Model file for the job. Use its own axes, mm. Round coordinates to 2 decimals unless told otherwise and drop trailing zeros. Loops run counter-clockwise (first coordinate to the right, second up) from the corner with the lowest first, then second, coordinate; pieces in that order, holes last.
from build123d import *

# Parameters (mm, degrees)
SKETCH1_R           = 60.5
SKETCH1_R_2         = 2.3
BOSS_EXTRUDE1_DEPTH = 2
SKETCH3_W           = 20
SKETCH3_H           = 4.8
CUT_EXTRUDE1_DEPTH  = 5
SKETCH4_W           = 165.999999998
SKETCH4_H           = 5
CUT_EXTRUDE2_DEPTH  = 5
SKETCH5_R           = 2.1
CUT_EXTRUDE3_DEPTH  = 5
SKETCH6_W           = 30
SKETCH6_H           = 2
SKETCH6_W_2         = 150
CUT_EXTRUDE4_DEPTH  = 5
SKETCH7_R           = 2.1
CUT_EXTRUDE5_DEPTH  = 5


with BuildPart() as part:
    # Sketch1 → Boss-Extrude1 (new body)
    with BuildSketch(Plane.XY):
        Polygon((125.000000001, -69.9), (75.000000001, -69.9), (75.000000001, -71.9), (55.000000001, -71.9), (55.000000001, -69.9), (-54.999999999, -69.9), (-54.999999999, -71.9), (-74.999999999, -71.9), (-74.999999999, -69.9), (-124.999999999, -69.9), (-124.999999999, -19.9), (-126.999999999, -19.9), (-126.999999999, 0.1), (-124.999999999, 0.1), (-124.999999999, 110.1), (-126.999999999, 110.1), (-126.999999999, 130.1), (-124.999999999, 130.1), (-124.999999999, 180.1), (125.000000001, 180.1), (125.000000001, 130.1), (127.000000001, 130.1), (127.000000001, 110.1), (125.000000001, 110.1), (125.000000001, 0.1), (127.000000001, 0.1), (127.000000001, -19.9), (125.000000001, -19.9), align=None)
        Circle(SKETCH1_R, mode=Mode.SUBTRACT)
        with Locations((0, -64)):
            Circle(SKETCH1_R_2, mode=Mode.SUBTRACT)
    extrude(amount=BOSS_EXTRUDE1_DEPTH)

    # Sketch3 → Cut-Extrude1 (cut)
    with BuildSketch(Plane.XY.offset(2)):
        with Locations((-102.999999999, 88.505234687)):
            Rectangle(SKETCH3_W, SKETCH3_H)
        with Locations((-102.999999999, 73.505234687)):
            Rectangle(SKETCH3_W, SKETCH3_H)
    cut_extrude1 = extrude(amount=-CUT_EXTRUDE1_DEPTH, mode=Mode.SUBTRACT)

    # Mirror1: Cut-Extrude1 across plane
    add(cut_extrude1.mirror(Plane(origin=(0, 0, 0), x_dir=(0, 0, 1), z_dir=(1, 0, 0))), mode=Mode.SUBTRACT)

    # Sketch4 → Cut-Extrude2 (cut)
    with BuildSketch(Plane.XY.offset(2)):
        with Locations((0, 88.505234687)):
            Rectangle(SKETCH4_W, SKETCH4_H)
        with Locations((0, 73.505234687)):
            Rectangle(SKETCH4_W, SKETCH4_H)
    extrude(amount=-CUT_EXTRUDE2_DEPTH, mode=Mode.SUBTRACT)

    # Sketch5 → Cut-Extrude3 (cut)
    with BuildSketch(Plane.XY.offset(2)):
        with Locations((-109.999999999, -54.9)):
            Circle(SKETCH5_R)
        with Locations((110.000000001, -54.9)):
            Circle(SKETCH5_R)
    extrude(amount=-CUT_EXTRUDE3_DEPTH, mode=Mode.SUBTRACT)

    # Sketch6 → Cut-Extrude4 (cut)
    with BuildSketch(Plane.XY.offset(2)):
        with Locations((-109.999999999, 179.1)):
            Rectangle(SKETCH6_W, SKETCH6_H)
        with Locations((1e-09, 179.1)):
            Rectangle(SKETCH6_W_2, SKETCH6_H)
        with Locations((110.000000001, 179.1)):
            Rectangle(SKETCH6_W, SKETCH6_H)
    extrude(amount=-CUT_EXTRUDE4_DEPTH, mode=Mode.SUBTRACT)

    # Sketch7 → Cut-Extrude5 (cut)
    with BuildSketch(Plane.XY.offset(2)):
        with Locations((-109.999999999, 163.1)):
            Circle(SKETCH7_R)
        with Locations((110.000000001, 163.1)):
            Circle(SKETCH7_R)
    extrude(amount=-CUT_EXTRUDE5_DEPTH, mode=Mode.SUBTRACT)


solid = part.part
Q1. Pull direction X, two halves, no side cores. Call faces 1 (the face through (-13.12, -59.06, 0.99)), 2 (the face through (2, 84, 2)): pulls with the +X half, pulls with the -X half, needs draft (parallel to the pull), parting line crosses it, or undercut.
Q2. Slice it at A-A on y = 9. Give the cut face in (x, z), plus the area to 3 significant figures.
Q3. Slice it at B-B on x = -10. Give the cut face in (y, z).
Q4. Slice it at D-D on y = 103.5. Give the cut face in (x, z), plus the area to 3 significant figures.
Q5. Probe line 1 (Y direction, x = -109.5, z = 0.2); line 2 (Y direction, x = 110, z = 1.05); line 3 (Y direction, x = 14.5, z = 1.2). List the from-to ranges inside material, lowest first.
Q6. Slice it at C-C on z = 1.5. State how many separate pieces and enclosed holes the cut face has, plus the area to 3 significant figures.
Q7. Flat gauge pins, fed straight in: P1, Ø5.5, axis at x = 110, y = -54.9, coming from the +Z side; P2, Ø1, axis at y = 179.5, z = 1.5, coming from the +X side; P3, Ø0.6, axis at y = 74, z = 1.5, coming from the -X side; P4, Ø0.6, axis at y = 72.5, z = 0.5, coming from the +X side. Where does each tip first touch, or does it go through?
Reply:
1. face 1: undercut
1. face 2: needs draft
2. outline: (-125, 0) - (-59.83, 0) - (-59.83, 2) - (-125, 2) - close; (59.83, 0) - (125, 0) - (125, 2) - (59.83, 2) - close
2. area: 261 mm2
3. outline: (-69.9, 0) - (-59.67, 0) - (-59.67, 2) - (-69.9, 2) - close; (59.67, 0) - (71.01, 0) - (71.01, 2) - (59.67, 2) - close; (76.01, 0) - (86.01, 0) - (86.01, 2) - (76.01, 2) - close; (91.01, 0) - (178.1, 0) - (178.1, 2) - (91.01, 2) - close
4. outline: (-125, 0) - (125, 0) - (125, 2) - (-125, 2) - close
4. area: 500 mm2
5. line 1: y = -69.9 to -56.94, -52.86 to 71.11, 75.91 to 86.11, 90.91 to 161.06, 165.14 to 178.1
5. line 2: y = -69.9 to -57, -52.8 to 71.11, 75.91 to 86.11, 90.91 to 161, 165.2 to 178.1
5. line 3: y = -69.9 to -58.74, 58.74 to 71.01, 76.01 to 86.01, 91.01 to 178.1
6. separate pieces: 1
6. enclosed holes: 12
6. area: 48,700 mm2
7. P1: stops at z = 2
7. P2: stops at x = 95
7. P3: stops at x = -125
7. P4: stops at x = 125
